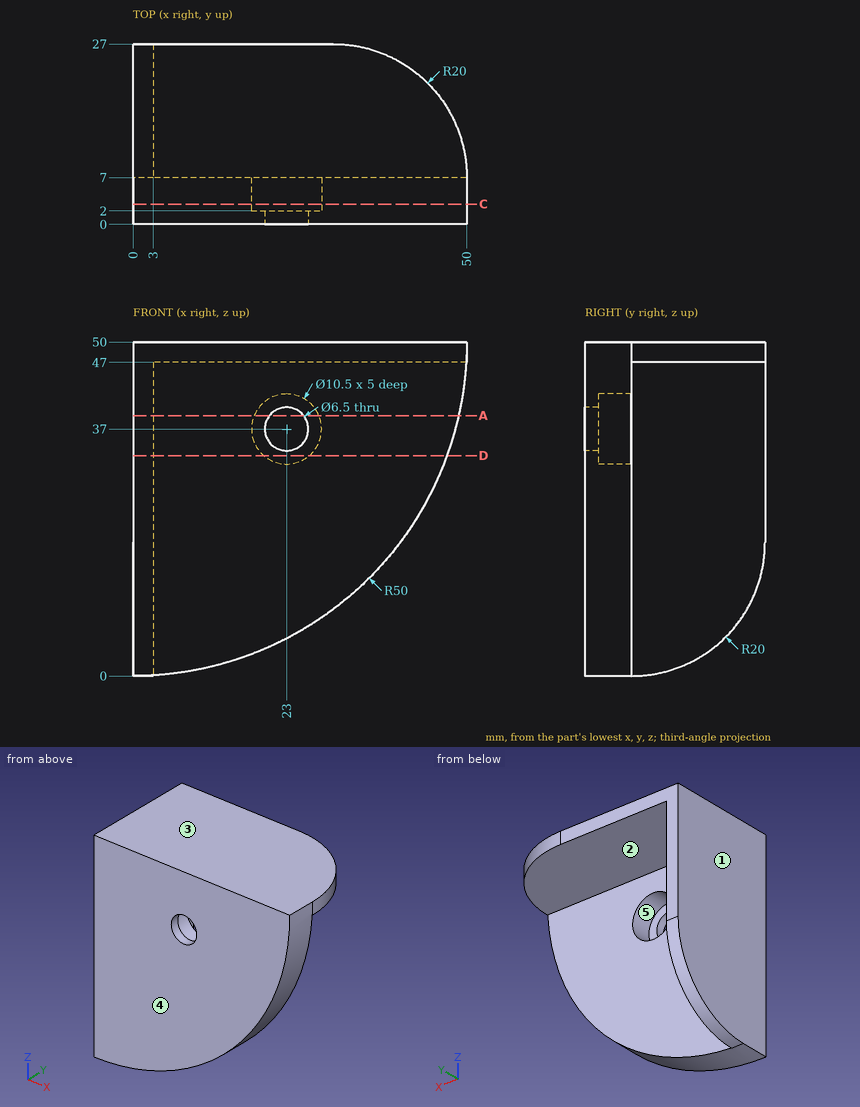
The figure shows three views and two pictorial views of one solid part (mm, origin at its lowest corner). Answer the questions. A direction names the side the tool comes from. Coordinates: 2 decimals unless noted, no trailing zeros. Write each loop counter-clockwise with the first axis right and the second up, starting at its lowest first coordinate (ties: lowest second). Pieces come first, ordered by that corner, then holes. Notation, with made-up numbers: (37, 18.5) -> (63, 18.5) arc R26 cw to (63, 51.5) -> close; hole circle Ø8 at (1, 16). An arc over 180 degrees is marked (long way). Return JSON: item names as keys, results as strings.
(1) The part is cut by section A-A on z = 39. Give the vertices of the cut face in (x, y) (1 decimal).
Answers below:
{"outline": "(0, 0) -> (20.4, 0) -> (20.4, 2) -> (18.1, 2) -> (18.1, 7) -> (3, 7) -> (3, 27) -> (0, 27) -> close; (25.6, 0) -> (48.8, 0) -> (48.8, 7) -> (27.9, 7) -> (27.9, 2) -> (25.6, 2) -> close"}
(2) Which of the six approach directions +Z, -Z, +X, -X, +Y, -Y give full straight-line access (tool end or side, diameter ignored) to the marked faces 1 and 2?
Answers below:
{"face 1": "+Z, -Z, -X, +Y, -Y", "face 2": "-Z, +X, +Y"}
(3) Each of these flat-tipped pins is pushed along its axis until it touches: P1, Ø5, axis at x = 22, z = 35.5, coming from the +Y side; P2, Ø3, axis at y = 8, z = 28, coming from the +X side; P3, Ø6, axis at x = 28.5, y = 14, coming from the -Z side; P4, Ø4, axis at x = 23, z = 37, coming from the +Y side. Where does it stop, or does it pass through?
Answers below:
{"P1": "y = 2", "P2": "x = 45.43", "P3": "z = 47", "P4": "through"}
(4) The part is cut by section D-D on z = 33. Give the vertices of the cut face in (x, y), then the cut area to 3 significant figures.
Answers below:
{"outline": "(0, 0) -> (47.02, 0) -> (47.02, 7) -> (26.4, 7) -> (26.4, 2) -> (19.6, 2) -> (19.6, 7) -> (3, 7) -> (3, 27) -> (0, 27) -> close", "area": "355 mm^2"}
(5) Consider line 1 along Z through (x, y) = (29.5, 23); line 2 along Y through (x, z) = (36, 45); line 3 along X through (y, z) = (10.5, 7). Determine where each line is inside the solid, lowest interval first. Write a range as from..to.
Answers below:
{"line 1": "47..50", "line 2": "0..7", "line 3": "0..3"}
(6) The part is cut by section C-C on y = 3. Give the vertices of the cut face in (x, z), then the cut area to 3 significant figures.
Answers below:
{"outline": "(0, 0) arc R50 ccw to (50, 50) -> (0, 50) -> close; hole circle Ø10.5 at (23, 37)", "area": "1,880 mm^2"}
(7) For a pull along Z with two mould halves and no side action, classify the marked faces 3, 4 and 5 as pulls with the +Z half, pulls with the -Z half, needs draft (parallel to the pull), parting line crosses it, or undercut.
Answers below:
{"face 3": "pulls with the +Z half", "face 4": "needs draft", "face 5": "undercut"}
